The model under review builds one solid part; all positions refer to its coordinate system, in mm. Face numbers are marked on the shaded views. A direction names the side the tool comes from. Round coordinates to 2 decimals unless told otherwise and drop trailing zeros. Write each loop counter-clockwise with the first axis right and the second up, starting at its lowest first coordinate (ties: lowest second). Pieces come first, ordered by that corner, then holes. Notation, with made-up numbers: (69, 70) -> (94, 70) arc R20 ccw to (94, 96) -> close; hole circle Ø3 at (65, 86.25). An arc over 180 degrees is marked (long way). Answer in a Markdown table with one row per item. Add a question column.
```python
from build123d import *

# Parameters (mm, degrees)
IZIM3_R                     = 15
Y_KSEKLIK_EKSTR_ZYON1_DEPTH = 20
IZIM4_R                     = 17.5
Y_KSEKLIK_EKSTR_ZYON2_DEPTH = 12.5


with BuildPart() as part:
    # Çizim3 → Yükseklik-Ekstrüzyon1 (new body)
    with BuildSketch(Plane.XY):
        Circle(IZIM3_R)
    extrude(amount=-Y_KSEKLIK_EKSTR_ZYON1_DEPTH)

    # Çizim4 → Yükseklik-Ekstrüzyon2 (add)
    with BuildSketch(Plane(origin=(0, 0, -20), x_dir=(-1, 0, 0), z_dir=(0, 0, -1))):
        Circle(IZIM4_R)
    extrude(amount=Y_KSEKLIK_EKSTR_ZYON2_DEPTH)

    # Çizim5 → Döndür4 (revolve)
    with BuildSketch(Plane(origin=(0, 0, 0), x_dir=(0, 0, -1), z_dir=(1, 0, 0))):
        with BuildLine():
            Line((50, 0), (32.5, 0))
            Line((32.5, 0), (32.5, -17.5))
            ThreePointArc((32.5, -17.5), (44.874368671, -12.374368671), (50, 0))
        make_face()
    revolve(axis=Axis((0, 0, -32.5), (0, 0, -1)))


solid = part.part
```
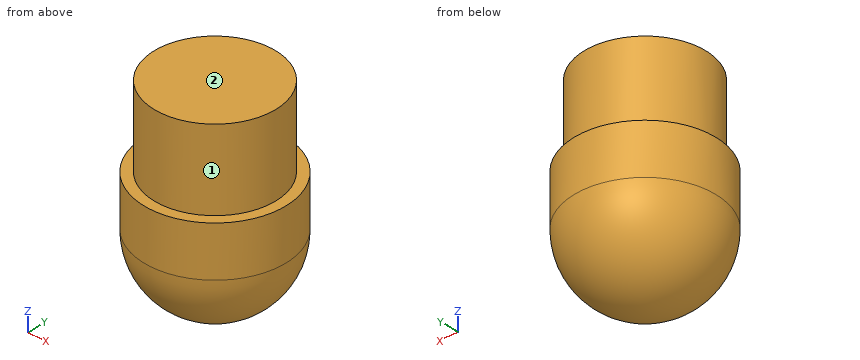
1. Add section A-A on x = 0. Write out the cut boundary in (y, z), plus the area to 3 significant figures.
2. For L1, parallel to Y at x = 0, z = -19.5; L2, parallel to X at y = -3, z = -18; L3, parallel to Y at x = 1.5, z = -10.5, list the stretches that pass through material, from the lowest coordinate up.
3. Insertion check: pin 1 Ø2 at (x, z) = (-8.5, -25.5) entering from +Y; pin 2 Ø1 at (x, y) = (11, -13.5) entering from +Z; pin 3 Ø1 at (x, z) = (-5, -15) entering from -Y. Each pin has a flat end and moves straight along its axis. Give the tip position at first contact, or say it passes through.
4. Tool access review of the marked faces 1 and 2: name each direction out of +Z, -Z, +X, -X, +Y, -Y from which nothing blocks a thin tool from reaching the whole face with its end or side.
5. Add section D-D on x = 3.5. Write out the cut boundary in (y, z), plus the area to 3 significant figures.
6. Add section C-C on z = -27.5. Write out the cut boundary in (x, y).
Filled in:
| question | item | result |
|---|---|---|
| 1 | outline | (-17.5, -32.5) arc R17.5 ccw to (17.5, -32.5) -> (17.5, -20) -> (15, -20) -> (15, 0) -> (-15, 0) -> (-15, -20) -> (-17.5, -20) -> close |
| 1 | area | 1,520 mm² |
| 2 | L1 | -15 to 15 |
| 2 | L2 | -14.7 to 14.7 |
| 2 | L3 | -14.92 to 14.92 |
| 3 | pin 1 | y = 15.81 |
| 3 | pin 2 | z = -20 |
| 3 | pin 3 | y = -14.31 |
| 4 | face 1 | +Z |
| 4 | face 2 | +Z, +X, -X, +Y, -Y |
| 5 | outline | (-17.15, -32.5) arc R17.15 ccw to (17.15, -32.5) -> (17.15, -20) -> (14.59, -20) -> (14.59, 0) -> (-14.59, 0) -> (-14.59, -20) -> (-17.15, -20) -> close |
| 5 | area | 1,470 mm² |
| 6 | outline | circle Ø35 at (0, 0) |
